Read the model definition and answer for the solid it produces. Units are mm, in the model's axes. Coordinates: 2 decimals unless noted, no trailing zeros. Write each loop counter-clockwise with the first axis right and the second up, starting at its lowest first coordinate (ties: lowest second). Pieces come first, ordered by that corner, then holes. Notation, with made-up numbers: (84.5, 47) -> (121.5, 47) arc R23 cw to (121.5, 61) -> close; hole circle Ø2 at (29.5, -20.5). An arc over 180 degrees is marked (long way). Write item = value, one per line. Start each with the question number.
1) Section B-B (x = 2.55) is taken. Determine the outline of the cut face in (y, z).
2) Section C-C (x = 1.2) is taken. Determine the outline of the cut face in (y, z).
3) Section A-A (y = 1) is taken. Determine the outline of the cut face in (x, z), plus the area to 3 significant figures.
4) Find the intervals of material crossed by line 1 along Z through (x, y) = (0, 1.05); line 2 along X through (y, z) = (0.9, 9); line 3 along Z through (x, y) = (-2.3, 1.25), in increasing order. Write a range as from..to.
5) For a pull along Y with two mould halves and no side action, classify faces 1 (the face through (0, 1.5, 0)), 2 (the face through (0, 1, 12)), 3 (the face through (0, 0, 0)) as released by +Y, released by -Y, zero draft, split by the parting line, or undercut.
Autodesk Inventor part; units mm, degrees
ref_plane "YZ Plane" through (0, 0, 0) normal (1, 0, 0) x (0, 1, 0)
ref_plane "XZ Plane" through (0, 0, 0) normal (0, 1, 0) x (-1, 0, 0)
ref_plane "XY Plane" through (0, 0, 0) normal (0, 0, 1) x (1, 0, 0)
sketch "Sketch1" plane through (0, 0, 0) normal (0, 1, 0) x (-1, 0, 0)
  line L0 (-3, -9) -> (3, -9)
  line L1 (3, -9) -> (3, 9)
  line L2 (3, 9) -> (-3, 9)
  line L3 (-3, 9) -> (-3, -9)
  line L4 (-3, -9) -> (3, 9) construction
  line L5 (3, -9) -> (-3, 9) construction
  circle A0 centre (0, -9) radius 3
  circle A1 centre (0, 9) radius 3
  point P0 (0, 0)
  dimension "d0" = 6
  dimension "d1" = 18
  dimension "d2" = 6
extrude "Extrusion1" add sketch "Sketch1" along normal blind 1.5
sketch "Sketch2" plane through (0, 1.5, 0) normal (0, 1, 0) x (1, 0, 0)
  arc A0 (-3, -9) -> (3, -9) centre (0, -9) ccw
  arc A1 (3, 9) -> (-3, 9) centre (0, 9) ccw
  circle A2 centre (0, 9) radius 1.5
  circle A3 centre (0, -9) radius 1.5
  point P0 (0, 0)
  dimension "d5" = 3
  dimension "d6" = 3
extrude "Extrusion2" cut sketch "Sketch2" against normal blind 2
sketch "Sketch7" plane through (0, 1.5, 0) normal (0, 1, 0) x (1, 0, 0)
  circle A0 centre (0, 9) radius 1.5
  circle A1 centre (0, -9) radius 1.5
  arc A2 (-3, -9) -> (3, -9) centre (0, -9) ccw
  arc A3 (3, 9) -> (-3, 9) centre (0, 9) ccw
  circle A4 centre (0, 9) radius 0.1
  circle A5 centre (0, -9) radius 0.1
  point P0 (0, 0)
  dimension "d13" = 0.2
  dimension "d14" = 0.2
extrude "Extrusion3" add sketch "Sketch7" against normal blind 1.5
properties part number "ruka_tahlo_sablona"
Answer key:
q1.outline = (0, -10.58) -> (1.5, -10.58) -> (1.5, 10.58) -> (0, 10.58) -> close
q2.outline = (0, -11.75) -> (1.5, -11.75) -> (1.5, 11.75) -> (0, 11.75) -> close
q3.outline = (-3, -9) arc R3 ccw to (3, -9) -> (3, 9) arc R3 ccw to (-3, 9) -> close; hole circle Ø0.2 at (0, -9); hole circle Ø0.2 at (0, 9)
q3.area = 136 mm^2
q4.line_1 = -12..-9.1, -8.9..8.9, 9.1..12
q4.line_2 = -3..-0.1, 0.1..3
q4.line_3 = -10.93..10.93
q5.face_1 = released by +Y
q5.face_2 = zero draft
q5.face_3 = released by -Y
